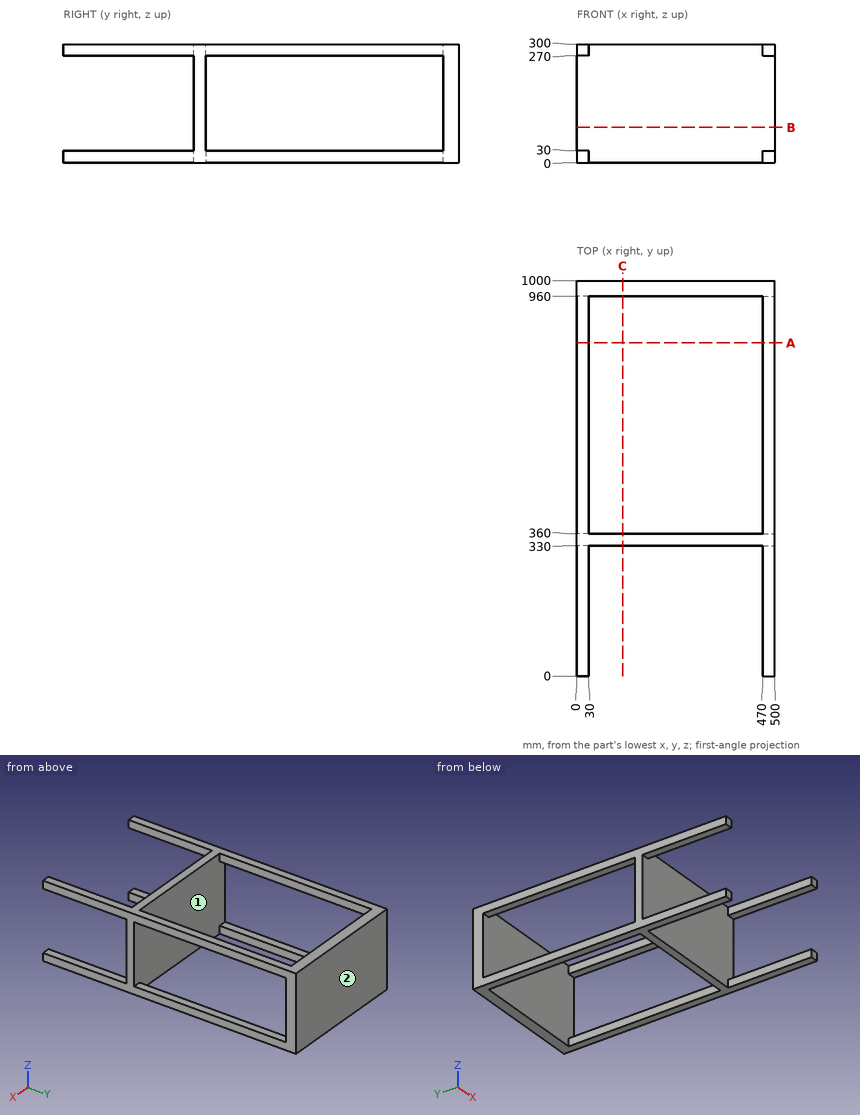
Input: dimensioned drawing with shaded views. Units: mm. Origin: part minimum x, y, z. Give positions to 0.01 mm unless a question says otherwise; leave off trailing zeros. Order: outer loops, then holes, each group sorted by start corner. A loop starts at its lowest first (then second) coordinate and runs counter-clockwise, first axis right, second up. Notation, with made-up numbers: (46, -1) -> (84, -1) arc R27 ccw to (84, 31) -> close; hole circle Ø1 at (42, 29). An arc over 180 degrees is marked (long way). Use one line per item in the form item = value.
1) Section B-B, the plane z = 89. Return loops of the section in (x, y), and give its area (3 significant figures).
Response values:
outline = (0, 330) -> (500, 330) -> (500, 360) -> (0, 360) -> close; (0, 960) -> (500, 960) -> (500, 1000) -> (0, 1000) -> close
area = 35,000 mm^2
2) Section C-C, the plane x = 116. Return loops of the section in (y, z).
Response values:
outline = (330, 0) -> (360, 0) -> (360, 300) -> (330, 300) -> close; (960, 0) -> (1000, 0) -> (1000, 300) -> (960, 300) -> close
3) Section A-A, the plane y = 842.5. Return loops of the section in (x, z), and give its area (3 significant figures).
Response values:
outline = (0, 0) -> (30, 0) -> (30, 30) -> (0, 30) -> close; (0, 270) -> (30, 270) -> (30, 300) -> (0, 300) -> close; (470, 0) -> (500, 0) -> (500, 30) -> (470, 30) -> close; (470, 270) -> (500, 270) -> (500, 300) -> (470, 300) -> close
area = 3,600 mm^2
4) Mould query, pull axis X, two halves, no side actions, for the marked faces 1 and 2. Classes: pulls with the +X half, pulls with the -X half, needs draft (parallel to the pull), parting line crosses it, or undercut.
Response values:
face_1 = undercut
face_2 = needs draft
5) First-contact query: pin 1 Ø1 at (x, z) = (388, 73.5) entering from -Y. Flat tip, straight axial feed; report the tip coordinate or a pass-through.
Response values:
pin_1 = 330
6) Line query: probe 1 along Y at (x, z) = (108, 194); probe 2 along X at (y, z) = (393, 274.5); probe 3 along Z at (x, y) = (23.5, 159). Output: solid intervals per line, ascending.
Response values:
probe_1 = 330 to 360, 960 to 1000
probe_2 = 0 to 30, 470 to 500
probe_3 = 0 to 30, 270 to 300
